The figure shows three views and two pictorial views of one solid part (mm, origin at its lowest corner). Answer the questions. Coordinates: 2 decimals unless noted, no trailing zeros. Write each loop counter-clockwise with the first axis right and the second up, starting at its lowest first coordinate (ties: lowest second). Pieces come first, ordered by that corner, then holes.
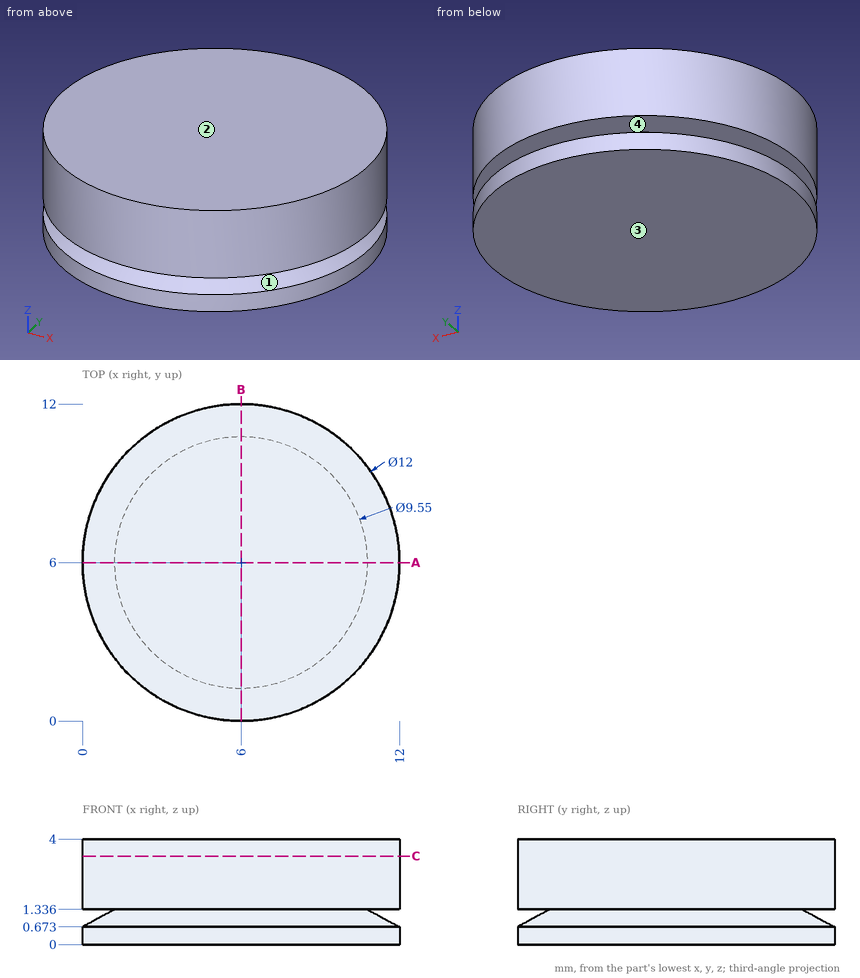
Q1. Given pin 1 (1 mm diameter, centred on x = 4.5, z = 1, fed in from +Y), flat-ended and moving along its own axis, determine where the tip first touches the part or whether it passes through.
Answers below:
pin 1: stops at y = 11.89
Q2. The part is cut by section C-C, the plane z = 3.35. Write down the section's boundary in (x, y), then the cut area to 3 significant figures.
Answers below:
outline: circle Ø12 at (6, 6)
area: 113 mm2
Q3. Find the intervals of material crossed by probe 1 along Z at (x, y) = (4.75, 1) (1 decimal); probe 2 along Z at (x, y) = (4.25, 1.25) (1 decimal); probe 3 along Y at (x, z) = (10, 3.8), in increasing order.
Answers below:
probe 1: z = 0 to 1.1, 1.3 to 4
probe 2: z = 0 to 1.2, 1.3 to 4
probe 3: y = 1.53 to 10.47
Q4. The part is cut by section A-A, the plane y = 6. Write down the section's boundary in (x, z) (1 decimal).
Answers below:
outline: (0, 0) - (12, 0) - (12, 0.7) - (10.8, 1.3) - (12, 1.3) - (12, 4) - (0, 4) - (0, 1.3) - (1.2, 1.3) - (0, 0.7) - close
Q5. Determine the mould class of the marked faces 1, 2, 3 and 4 for opening direction Z: released by +Z, released by -Z, zero draft, split by the parting line, or undercut.
Answers below:
face 1: undercut
face 2: released by +Z
face 3: released by -Z
face 4: undercut
